Input: dimensioned drawing with shaded views. Units: mm. Origin: part minimum x, y, z. A direction names the side the tool comes from. Give positions to 0.01 mm unless a question says otherwise; leave off trailing zeros. Write each loop counter-clockwise with the first axis right and the second up, starting at its lowest first coordinate (ties: lowest second). Pieces come first, ordered by that corner, then holes.
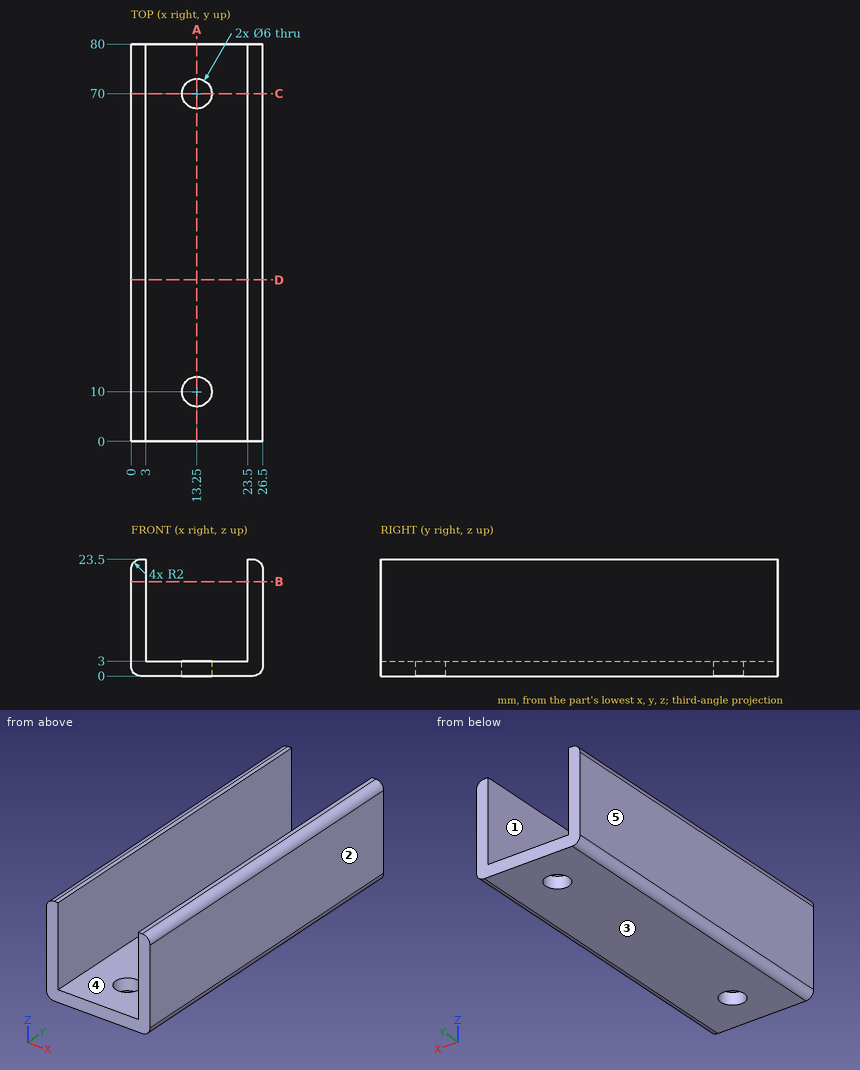
Item 1: Pin query (flat end, axial travel): pin 1 Ø5 at (x, y) = (17, 34.5) entering from +Z. Return the tip coordinate at first contact, or that it passes through.
Found:
pin 1: stops at z = 3
Item 2: Section B-B, the plane z = 19. Return the cut outline in (x, y).
Found:
outline: (0, 0) - (3, 0) - (3, 80) - (0, 80) - close; (23.5, 0) - (26.5, 0) - (26.5, 80) - (23.5, 80) - close
Item 3: Section C-C, the plane y = 70. Return the cut outline in (x, z), plus the area to 3 significant figures.
Found:
outline: (0, 2) arc R2 ccw to (2, 0) - (10.25, 0) - (10.25, 3) - (3, 3) - (3, 23.5) - (2, 23.5) arc R2 ccw to (0, 21.5) - close; (16.25, 0) - (24.5, 0) arc R2 ccw to (26.5, 2) - (26.5, 21.5) arc R2 ccw to (24.5, 23.5) - (23.5, 23.5) - (23.5, 3) - (16.25, 3) - close
area: 181 mm2
Item 4: Pull-direction query (X, two-part tool) for the marked faces 1, 2 and 3; classes: +X half, -X half, draft (parallel to the pull), parting line (faces both ways), or undercut.
Found:
face 1: undercut
face 2: +X half
face 3: draft
Item 5: Reachability of the marked faces 4 and 5 from +Z, -Z, +X, -X, +Y, -Y: full face, straight path, thin tool, end or side. Return the list, or none.
Found:
face 4: +Z, +Y, -Y
face 5: +Z, -Z, -X, +Y, -Y
Item 6: Line query: L1, parallel to Y at x = 13.25, z = 1.8; L2, parallel to X at y = 57, z = 4.75; L3, parallel to Z at x = 11.75, y = 28.5. Output: solid intervals per line, ascending.
Found:
L1: y = 0 to 7, 13 to 67, 73 to 80
L2: x = 0 to 3, 23.5 to 26.5
L3: z = 0 to 3
Item 7: Section D-D, the plane y = 32.5. Return the cut outline in (x, z), plus the area to 3 significant figures.
Found:
outline: (0, 2) arc R2 ccw to (2, 0) - (24.5, 0) arc R2 ccw to (26.5, 2) - (26.5, 21.5) arc R2 ccw to (24.5, 23.5) - (23.5, 23.5) - (23.5, 3) - (3, 3) - (3, 23.5) - (2, 23.5) arc R2 ccw to (0, 21.5) - close
area: 199 mm2
Item 8: Section A-A, the plane x = 13.25. Return the cut outline in (y, z).
Found:
outline: (0, 0) - (7, 0) - (7, 3) - (0, 3) - close; (13, 0) - (67, 0) - (67, 3) - (13, 3) - close; (73, 0) - (80, 0) - (80, 3) - (73, 3) - close
